For this review, take the finished solid that the model builds, in its own axes (mm). Face numbers are marked on the shaded views. A direction names the side the tool comes from. Give positions to 0.01 mm unless a question says otherwise; leave off trailing zeros. Write each loop counter-clockwise with the first axis right and the second up, starting at its lowest first coordinate (ties: lowest second). Pieces come first, ordered by that corner, then holes.
Q1. For line 1 (X direction, y = -5.5, z = 1.75); line 2 (Y direction, x = -46.35, z = 6); line 3 (Z direction, x = -45.8, y = -0.5), list the stretches that pass through material, from the lowest coordinate up.
Q2. Mouldability with a two-part tool opening along X and no side actions: class the marked faces 1, 2 and 3 as released by +X, released by -X, zero draft, split by the parting line, or undercut.
Q3. Machinability: for the marked faces 4, 5 and 6, which of the approach directions +Z, -Z, +X, -X, +Y, -Y give a long, thin tool a straight path to every point of the face, cutting with its end or side? Answer none if there is none.
Q4. We need section D-D (z = 6). Write out the cut boundary in (x, y), then the cut area to 3 significant figures.
Q5. We need section A-A (x = -83). Write out the cut boundary in (y, z).
Q6. We need section B-B (y = -0.5). Write out the cut boundary in (x, z), then the cut area to 3 significant figures.
Q7. We need section C-C (z = 1). Write out the cut boundary in (x, y), then the cut area to 3 significant figures.
Q8. Insertion check: P1, Ø1, axis at x = -59, y = 0, coming from the -Z side; P2, Ø1.5, axis at x = -59, z = 5, coming from the -Y side (3 decimals); P3, Ø2, axis at x = -59.5, y = 6.5, coming from the +Z side; P4, Ø3, axis at x = -63, y = -8, coming from the +Z side. Each pin has a flat end and moves straight along its axis. Give the tip position at first contact, or say it passes through.
```python
from build123d import *

# Parameters (mm, degrees)
CYLINDER032_R           = 1.4
CYLINDER032_DEPTH       = 5
CYLINDER033_R           = 1.4
CYLINDER033_DEPTH       = 5
BOX046_W                = 8
BOX046_H                = 12
BOX046_DEPTH            = 10
BOX045_W                = 8
BOX045_H                = 12
BOX045_DEPTH            = 10
CYLINDER031_R           = 1.5
CYLINDER031_DEPTH       = 10
CYLINDER031_PITCH_ANGLE = 90
BOX044_W                = 3
BOX044_H                = 32
BOX044_DEPTH            = 13
BOX043_W                = 48
BOX043_H                = 32
BOX043_DEPTH            = 3


with BuildPart() as cilindro032:
    # Cylinder032 → Cylinder032 (new body)
    with BuildSketch(Plane(origin=(-63, 6, 3), x_dir=(1, 0, 0), z_dir=(0, 0, 1))):
        Circle(CYLINDER032_R)
    extrude(amount=CYLINDER032_DEPTH)


with BuildPart() as cilindro033:
    # Cylinder033 → Cylinder033 (new body)
    with BuildSketch(Plane(origin=(-63, -8, 3), x_dir=(1, 0, 0), z_dir=(0, 0, 1))):
        Circle(CYLINDER033_R)
    extrude(amount=CYLINDER033_DEPTH)


with BuildPart() as cubo040:
    # Box046 → Box046 (new body)
    with BuildSketch(Plane(origin=(-89, 0, -2), x_dir=(1, 0, 0), z_dir=(0, 0, 1))):
        with Locations((4, 6)):
            Rectangle(BOX046_W, BOX046_H)
    extrude(amount=BOX046_DEPTH)


with BuildPart() as cubo039:
    # Box045 → Box045 (new body)
    with BuildSketch(Plane(origin=(-89, -14, -2), x_dir=(1, 0, 0), z_dir=(0, 0, 1))):
        with Locations((4, 6)):
            Rectangle(BOX045_W, BOX045_H)
    extrude(amount=BOX045_DEPTH)


with BuildPart() as cilindro031:
    # Cylinder031 → Cylinder031 (new body)
    with BuildSketch(Plane.XY):
        Circle(CYLINDER031_R)
    extrude(amount=CYLINDER031_DEPTH)


with BuildPart() as cilindro031_1:
    # Cylinder031 pitch: moved
    add(cilindro031.part.rotate(Axis((0, 0, 0), (0, 1, 0)), CYLINDER031_PITCH_ANGLE))


with BuildPart() as cilindro031_2:
    # Cylinder031 placement: moved
    add(cilindro031_1.part.moved(Location((-51, -0.5, 6))))


with BuildPart() as cubo038:
    # Box044 → Box044 (new body)
    with BuildSketch(Plane(origin=(-48, -17, 0), x_dir=(1, 0, 0), z_dir=(0, 0, 1))):
        with Locations((1.5, 16)):
            Rectangle(BOX044_W, BOX044_H)
    extrude(amount=BOX044_DEPTH)


with BuildPart() as obj1:
    # Box043 → Box043 (new body)
    with BuildSketch(Plane(origin=(-93, -17, 0), x_dir=(1, 0, 0), z_dir=(0, 0, 1))):
        with Locations((24, 16)):
            Rectangle(BOX043_W, BOX043_H)
    extrude(amount=BOX043_DEPTH)

    # Fusion013: union Cubo038
    add(cubo038.part)

    # Cut056: cut Cilindro031
    add(cilindro031_2.part, mode=Mode.SUBTRACT)

    # Cut057: cut Cubo039
    add(cubo039.part, mode=Mode.SUBTRACT)

    # Cut058: cut Cubo040
    add(cubo040.part, mode=Mode.SUBTRACT)

    # Fusion014: union Cilindro032, Cilindro033
    add(cilindro032.part)
    add(cilindro033.part)


solid = obj1.part
```
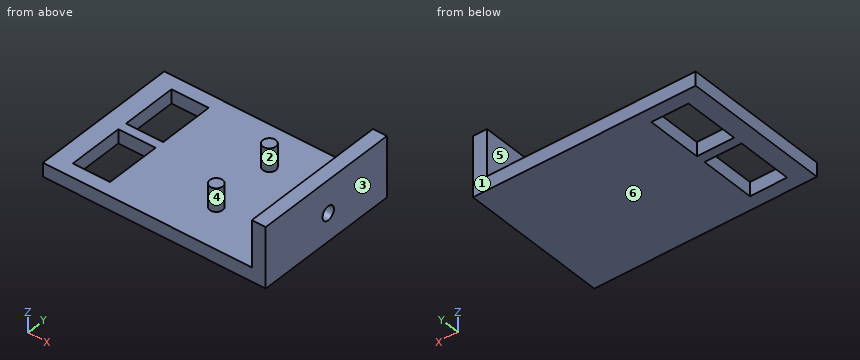
Computed:
1. line 1: x = -93 to -89, -81 to -45
1. line 2: y = -17 to -2, 1 to 15
1. line 3: z = 0 to 4.5, 7.5 to 13
2. face 1: zero draft
2. face 2: undercut
2. face 3: released by +X
3. face 4: +Z
3. face 5: +Z, +Y, -Y
3. face 6: -Z, +X, -X, +Y, -Y
4. outline: circle Ø2.8 at (-63, -8); circle Ø2.8 at (-63, 6); (-48, -17) - (-45, -17) - (-45, -2) - (-48, -2) - close; (-48, 1) - (-45, 1) - (-45, 15) - (-48, 15) - close
4. area: 99.3 mm2
5. outline: (-17, 0) - (-14, 0) - (-14, 3) - (-17, 3) - close; (-2, 0) - (0, 0) - (0, 3) - (-2, 3) - close; (12, 0) - (15, 0) - (15, 3) - (12, 3) - close
6. outline: (-93, 0) - (-45, 0) - (-45, 4.5) - (-48, 4.5) - (-48, 3) - (-93, 3) - close; (-48, 7.5) - (-45, 7.5) - (-45, 13) - (-48, 13) - close
6. area: 165 mm2
7. outline: (-93, -17) - (-45, -17) - (-45, 15) - (-93, 15) - close; hole (-89, -14) - (-81, -14) - (-81, -2) - (-89, -2) - close; hole (-89, 0) - (-81, 0) - (-81, 12) - (-89, 12) - close
7. area: 1,340 mm2
8. P1: stops at z = 0
8. P2: passes through
8. P3: stops at z = 3
8. P4: stops at z = 8
